Read the model definition and answer for the solid it produces. Units are mm, in the model's axes. A direction names the side the tool comes from. Give positions to 0.01 mm unless a question says otherwise; leave off trailing zeros. Order: outer loops, then holes, each group sorted by start corner. A loop starts at its lowest first (then second) coordinate and runs counter-clockwise, first axis right, second up. Notation, with made-up numbers: (-13, 78) -> (35, 78) arc R9 cw to (35, 90) -> close; hole circle Ø6 at (36, 46). An arc over 180 degrees is marked (long way). One line per question, with ' | ' between items. Start each with the question number.
```python
from build123d import *

# Parameters (mm, degrees)
SKETCH1_W                            = 254
SKETCH1_H                            = 57.15
SKETCH1_R                            = 10
BOSS_EXTRUDE1_DEPTH                  = 6.730000002
SKETCH25_R                           = 10.25
CUT_EXTRUDE1_DEPTH                   = 7.6
SKETCH26_W                           = 254
SKETCH26_H                           = 57.15
BOSS_EXTRUDE2_DEPTH                  = 0.4
F_11_64_0_17188_DIAMETER_HOLE1_D     = 4.365752
F_11_64_0_17188_DIAMETER_HOLE1_DEPTH = 6.35
F_11_64_0_17188_DIAMETER_HOLE1_TIP   = 1.311604225
F_11_64_0_17188_DIAMETER_HOLE2_D     = 4.365752
F_11_64_0_17188_DIAMETER_HOLE2_DEPTH = 6.35
F_11_64_0_17188_DIAMETER_HOLE2_TIP   = 1.311604225


with BuildPart() as part:
    # Sketch1 → Boss-Extrude1 (new body)
    with BuildSketch(Plane(origin=(0, 0, 0), x_dir=(1, 0, 0), z_dir=(0, 1, 0))):
        with Locations((92.969183673, -14.086632653)):
            Rectangle(SKETCH1_W, SKETCH1_H)
        with Locations(Location((202.969183673, 0.518367347, 0), (0, 0, 270))):
            Circle(SKETCH1_R, mode=Mode.SUBTRACT)
        with Locations(Location((171.219183673, 0.518367347, 0), (0, 0, 270))):
            Circle(SKETCH1_R, mode=Mode.SUBTRACT)
        with Locations(Location((139.469183673, 0.518367347, 0), (0, 0, 270))):
            Circle(SKETCH1_R, mode=Mode.SUBTRACT)
        with Locations(Location((107.719183673, 0.518367347, 0), (0, 0, 270))):
            Circle(SKETCH1_R, mode=Mode.SUBTRACT)
        with Locations(Location((75.969183673, 0.518367347, 0), (0, 0, 270))):
            Circle(SKETCH1_R, mode=Mode.SUBTRACT)
        with Locations(Location((44.219183673, 0.518367347, 0), (0, 0, 270))):
            Circle(SKETCH1_R, mode=Mode.SUBTRACT)
        with Locations(Location((171.219183673, -22.341632653, 0), (0, 0, 270))):
            Circle(SKETCH1_R, mode=Mode.SUBTRACT)
        with Locations(Location((139.469183673, -22.341632653, 0), (0, 0, 270))):
            Circle(SKETCH1_R, mode=Mode.SUBTRACT)
        with Locations(Location((107.719183673, -22.341632653, 0), (0, 0, 270))):
            Circle(SKETCH1_R, mode=Mode.SUBTRACT)
        with Locations(Location((75.969183673, -22.341632653, 0), (0, 0, 270))):
            Circle(SKETCH1_R, mode=Mode.SUBTRACT)
        with Locations(Location((44.219183673, -22.341632653, 0), (0, 0, 270))):
            Circle(SKETCH1_R, mode=Mode.SUBTRACT)
        with Locations(Location((202.969183673, -22.341632653, 0), (0, 0, 270))):
            Circle(SKETCH1_R, mode=Mode.SUBTRACT)
        with Locations(Location((12.469183673, 0.518367347, 0), (0, 0, 270))):
            Circle(SKETCH1_R, mode=Mode.SUBTRACT)
        with Locations(Location((-19.280816327, 0.518367347, 0), (0, 0, 270))):
            Circle(SKETCH1_R, mode=Mode.SUBTRACT)
        with Locations(Location((12.469183673, -22.341632653, 0), (0, 0, 270))):
            Circle(SKETCH1_R, mode=Mode.SUBTRACT)
        with Locations(Location((-19.280816327, -22.341632653, 0), (0, 0, 270))):
            Circle(SKETCH1_R, mode=Mode.SUBTRACT)
    extrude(amount=BOSS_EXTRUDE1_DEPTH)

    # Sketch25 → Cut-Extrude1 (cut)
    with BuildSketch(Plane.XZ):
        with Locations(Location((44.219183673, 22.341632653, 0), (0, 0, 270))):
            Circle(SKETCH25_R)
        with Locations(Location((75.969183673, 22.341632653, 0), (0, 0, 270))):
            Circle(SKETCH25_R)
        with Locations(Location((107.719183673, 22.341632653, 0), (0, 0, 270))):
            Circle(SKETCH25_R)
        with Locations(Location((139.469183673, 22.341632653, 0), (0, 0, 270))):
            Circle(SKETCH25_R)
        with Locations(Location((171.219183673, 22.341632653, 0), (0, 0, 270))):
            Circle(SKETCH25_R)
        with Locations(Location((202.969183673, 22.341632653, 0), (0, 0, 270))):
            Circle(SKETCH25_R)
        with Locations(Location((75.969183673, -0.518367347, 0), (0, 0, 270))):
            Circle(SKETCH25_R)
        with Locations(Location((107.719183673, -0.518367347, 0), (0, 0, 270))):
            Circle(SKETCH25_R)
        with Locations(Location((139.469183673, -0.518367347, 0), (0, 0, 270))):
            Circle(SKETCH25_R)
        with Locations(Location((171.219183673, -0.518367347, 0), (0, 0, 270))):
            Circle(SKETCH25_R)
        with Locations(Location((202.969183673, -0.518367347, 0), (0, 0, 270))):
            Circle(SKETCH25_R)
        with Locations(Location((44.219183673, -0.518367347, 0), (0, 0, 270))):
            Circle(SKETCH25_R)
        with Locations(Location((12.469183673, 22.341632653, 0), (0, 0, 270))):
            Circle(SKETCH25_R)
        with Locations(Location((-19.280816327, 22.341632653, 0), (0, 0, 270))):
            Circle(SKETCH25_R)
        with Locations(Location((-19.280816327, -0.518367347, 0), (0, 0, 270))):
            Circle(SKETCH25_R)
        with Locations(Location((12.469183673, -0.518367347, 0), (0, 0, 270))):
            Circle(SKETCH25_R)
    extrude(amount=-CUT_EXTRUDE1_DEPTH, mode=Mode.SUBTRACT)

    # Sketch26 → Boss-Extrude2 (add)
    with BuildSketch(Plane(origin=(0, 6.730000002, 0), x_dir=(1, 0, 0), z_dir=(0, 1, 0))):
        with Locations((92.969183673, -14.086632653)):
            Rectangle(SKETCH26_W, SKETCH26_H)
    extrude(amount=-BOSS_EXTRUDE2_DEPTH)

    # 11/64 (0.17188) Diameter Hole1
    with Locations(Plane.XY.offset(42.661632653)):
        with Locations((21.849183673, 4.064), (148.849183673, 4.064), (85.349183673, 4.064)):
            Hole(F_11_64_0_17188_DIAMETER_HOLE1_D / 2, depth=F_11_64_0_17188_DIAMETER_HOLE1_DEPTH)
            with Locations((0, 0, -(F_11_64_0_17188_DIAMETER_HOLE1_DEPTH + F_11_64_0_17188_DIAMETER_HOLE1_TIP / 2))):  # 118° drill point
                Cone(0, F_11_64_0_17188_DIAMETER_HOLE1_D / 2, F_11_64_0_17188_DIAMETER_HOLE1_TIP, mode=Mode.SUBTRACT)

    # 11/64 (0.17188) Diameter Hole2
    with Locations(Plane(origin=(0, 0, -14.488367347), x_dir=(-1, 0, 0), z_dir=(0, 0, -1))):
        with Locations((-148.849183673, 4.064), (-85.349183673, 4.064), (-21.849183673, 4.064)):
            Hole(F_11_64_0_17188_DIAMETER_HOLE2_D / 2, depth=F_11_64_0_17188_DIAMETER_HOLE2_DEPTH)
            with Locations((0, 0, -(F_11_64_0_17188_DIAMETER_HOLE2_DEPTH + F_11_64_0_17188_DIAMETER_HOLE2_TIP / 2))):  # 118° drill point
                Cone(0, F_11_64_0_17188_DIAMETER_HOLE2_D / 2, F_11_64_0_17188_DIAMETER_HOLE2_TIP, mode=Mode.SUBTRACT)


solid = part.part
```
Q1. Which of the six approach directions +Z, -Z, +X, -X, +Y, -Y give full straight-line access (tool end or side, diameter ignored) to faces 4 (the cylindrical face through (19.767, 4.72, 39.442)), 5 (the cylindrical face through (19.67, 4.16, -11.27)), 6 (the cylindrical face through (116.36, 3.12, 16.83))?
Q2. Determine the mould class of faces 1 (the cylindrical face through (-16.202, 3.121, -10.295)), 2 (the cylindrical face through (66.876, 3.121, 17.612)), 3 (the flat face through (-34.031, 3, 14)) for opening direction X: pulls with the +X half, pulls with the -X half, needs draft (parallel to the pull), parting line crosses it, or undercut.
Q3. Given P1, Ø16.5, axis at x = 109.5, z = 26.5, coming from the -Y side; P2, Ø10, axis at x = 12, z = 24.5, coming from the -Y side; P3, Ø2.5, axis at x = 148.85, y = 4.06, coming from the -Z side; P4, Ø3.5, axis at x = 85.35, y = 4.06, coming from the -Z side, each flat-ended and moving along its own axis, determine where each tip first touches the part or whether it passes through.
Q4. Find the intervals of material crossed by line 1 (Z direction, x = 140, y = 5); line 2 (Z direction, x = 67, y = 5.5); line 3 (Y direction, x = 162.5, z = -3), in increasing order.
Q5. A cutting plane is placed at B-B, the plane y = 3. Give the number of separate pieces and of enclosed holes in the cut face, then the cut area to 3 significant figures.
Q6. A cutting plane is placed at C-C, the plane x = 6. Determine the outline of the cut face in (y, z).
Q7. A cutting plane is placed at A-A, the plane x = 197. Determine the outline of the cut face in (y, z), then the cut area to 3 significant figures.
Geometry results:
1) face 4: +Z | face 5: -Z | face 6: -Y
2) face 1: undercut | face 2: undercut | face 3: pulls with the -X half
3) P1: y = 0 | P2: y = 6.33 | P3: z = -7.58 | P4: z = -7.88
4) line 1: -14.49 to -10.75, 9.72 to 12.11, 32.58 to 42.66 | line 2: -14.49 to -5.48, 4.44 to 17.38, 27.3 to 42.66 | line 3: 6.33 to 6.73
5) separate pieces: 1 | enclosed holes: 16 | area: 9,080 mm²
6) outline: (0, -14.49) -> (6.73, -14.49) -> (6.73, 42.66) -> (0, 42.66) -> (0, 30.29) -> (6.33, 30.29) -> (6.33, 14.39) -> (0, 14.39) -> (0, 7.43) -> (6.33, 7.43) -> (6.33, -8.47) -> (0, -8.47) -> close
7) outline: (0, -14.49) -> (6.73, -14.49) -> (6.73, 42.66) -> (0, 42.66) -> (0, 30.67) -> (6.33, 30.67) -> (6.33, 14.01) -> (0, 14.01) -> (0, 7.81) -> (6.33, 7.81) -> (6.33, -8.85) -> (0, -8.85) -> close | area: 174 mm²
